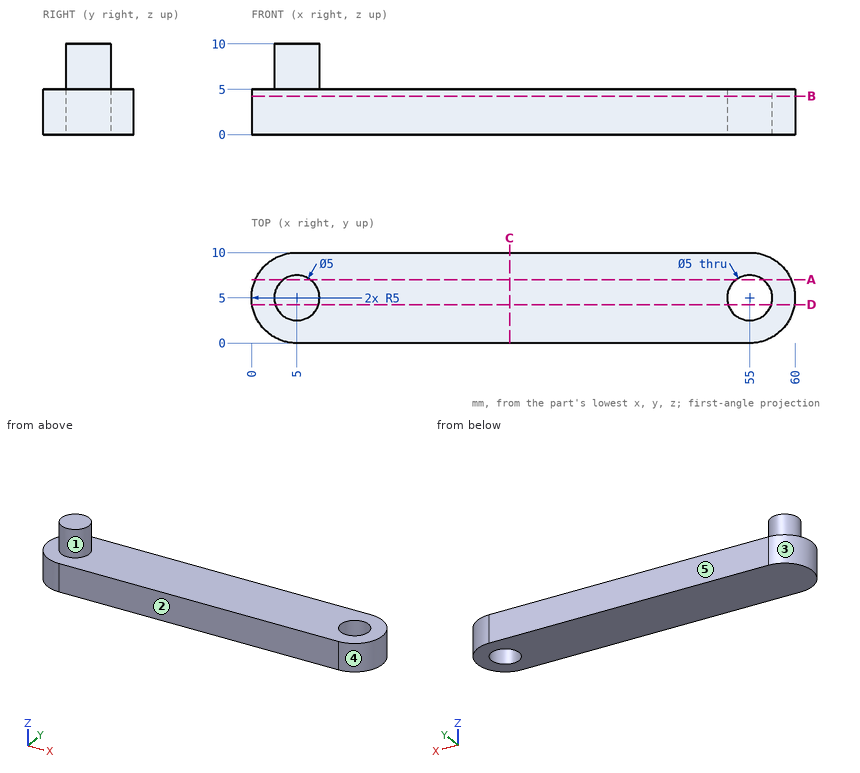
Part print with two shaded views. Sizes in mm from the minimum x, y, z corner. A direction names the side the tool comes from. Round coordinates to 2 decimals unless told otherwise and drop trailing zeros. Write each loop counter-clockwise with the first axis right and the second up, starting at its lowest first coordinate (ties: lowest second). Pieces come first, ordered by that corner, then holes. Notation, with made-up numbers: M 22,75.25 L 72,75.25 A20 ccw 72,104.25 Z; hole C -15.5,70.5 d3. An arc over 180 degrees is marked long. Answer as CSV lines item,"result". Start each with the question number.
1) Which spindle directions (+Z, -Z, +X, -X, +Y, -Y) get a long thin tool onto all of the face, cutting with end or side? Do the marked faces 1 and 2. Say none if no direction does.
2) Band-saw the part on A-A (y = 7). List the corners of the cut face in (x, z).
3) Band-saw the part on D-D (y = 4.25). List the corners of the cut face in (x, z), then the cut area to 3 significant figures.
4) Band-saw the part on B-B (z = 4.25). List the corners of the cut face in (x, y), then the cut area to 3 significant figures.
5) Mould opens along X. For the marked faces 3, 4 and 5 say: +X half, -X half, draft (parallel to the pull), parting line (faces both ways), or undercut.
6) Band-saw the part on C-C (x = 28.5). List the corners of the cut face in (y, z), then the cut area to 3 significant figures.
7) Drill centre lines: L1, parallel to Y at x = 55, z = 2.95; L2, parallel to X at y = 5.25, z = 8.5; L3, parallel to X at y = 6.75, z = 4.5. Where is each one in solid material? Low to high.
8) Drop flat-ended pins along their axis: pin 1 (3 mm diameter, centred on x = 55, y = 5, fed in from -Z); pin 2 (4 mm diameter, centred on y = 6.5, z = 8, fed in from -X); pin 3 (1.5 mm diameter, centred on y = 3.5, z = 4, fed in from -X). Give the stop position or say it passes through.
Worked out:
1,face 1,"+Z"
1,face 2,"+Z, -Z, +X, -X, -Y"
2,outline,"M 0.42,0 L 53.5,0 L 53.5,5 L 6.5,5 L 6.5,10 L 3.5,10 L 3.5,5 L 0.42,5 Z; M 56.5,0 L 59.58,0 L 59.58,5 L 56.5,5 Z"
3,outline,"M 0.06,0 L 52.62,0 L 52.62,5 L 7.38,5 L 7.38,10 L 2.62,10 L 2.62,5 L 0.06,5 Z; M 57.38,0 L 59.94,0 L 59.94,5 L 57.38,5 Z"
3,area,"299 mm²"
4,outline,"M 5,0 L 55,0 A5 ccw 55,10 L 5,10 A5 ccw Z; hole C 55,5 d5"
4,area,"559 mm²"
5,face 3,"-X half"
5,face 4,"+X half"
5,face 5,"draft"
6,outline,"M 0,0 L 10,0 L 10,5 L 0,5 Z"
6,area,"50.0 mm²"
7,L1,"0 to 2.5, 7.5 to 10"
7,L2,"2.51 to 7.49"
7,L3,"0.32 to 53.21, 56.79 to 59.68"
8,pin 1,"through"
8,pin 2,"x = 2.5"
8,pin 3,"x = 0.06"
